```python
from build123d import *

# Parameters (mm, degrees)
SKETCH1_R           = 73.66
BOSS_EXTRUDE1_DEPTH = 0.635
BOSS_EXTRUDE2_START = 52.324
SKETCH2_R           = 73.66
SKETCH2_R_2         = 73.025
BOSS_EXTRUDE2_DEPTH = 52.324
FILLET1_R           = 2.54


with BuildPart() as part:
    # Sketch1 → Boss-Extrude1 (new body)
    with BuildSketch(Plane.XY):
        Circle(SKETCH1_R)
    extrude(amount=BOSS_EXTRUDE1_DEPTH)

    # Sketch2 → Boss-Extrude2 (add)
    with BuildSketch(Plane(origin=(0, 0, 0), x_dir=(-1, 0, 0), z_dir=(0, 0, -1)).offset(BOSS_EXTRUDE2_START)):
        Circle(SKETCH2_R)
        Circle(SKETCH2_R_2, mode=Mode.SUBTRACT)
    extrude(amount=-BOSS_EXTRUDE2_DEPTH)

    # Fillet1
    fillet1_edges = [part.edges().sort_by_distance(p)[0] for p in [
        (-73.66, 0, 0.635),
    ]]
    fillet(fillet1_edges, radius=FILLET1_R)


solid = part.part
```
The listing builds one solid part. Answer for the finished solid, in the listing's coordinates (mm). A direction names the side the tool comes from. Round coordinates to 2 decimals unless told otherwise and drop trailing zeros. Order: outer loops, then holes, each group sorted by start corner. A loop starts at its lowest first (then second) coordinate and runs counter-clockwise, first axis right, second up. Notation, with made-up numbers: (-18, 54) -> (32, 54) arc R15 cw to (32, 65) -> close; hole circle Ø9 at (-39.75, 34). An arc over 180 degrees is marked (long way). Answer as CSV lines item,"result". Start each with the question number.
(1) For a pull along Y with two mould halves and no side action, classify faces 3 (the face through (-1, 1, 0)), 4 (the face through (-1, 1, 0.635)), 5 (the face through (58.454, -44.821, -27.467)) as +Y half, -Y half, draft (parallel to the pull), parting line (faces both ways), or undercut.
(2) Flat-ended cylindrical pins translate along their axes: pin 1 Ø2 at (x, z) = (-42.5, -17.5) entering from -Y; pin 2 Ø4 at (y, z) = (55.5, -38) entering from +X; pin 3 Ø1.5 at (x, z) = (0.5, -45) entering from +Y. Find the tip coordinate at first contact, or state that the pin passes through.
(3) The part is cut by section A-A (z = -26). Determine the outline of the cut face in (x, y) (3 decimals), then the cut area to 3 significant figures.
(4) A tool of negligible diameter and unlimited length cuts with its end or side. For faces 1 (the face through (16.7, 71.3, -52.324)), 2 (the face through (-69.653, 21.935, -26.528)), from which of +Z, -Z, +X, -X, +Y, -Y can it reach the whole face along a straight path? Write none if from no direction.
(5) Find the intervals of material crossed by probe 1 along Y at (x, z) = (0, -33.5) (3 decimals); probe 2 along Z at (x, y) = (22, -33) (3 decimals); probe 3 along X at (y, z) = (-41.5, -19.5), in increasing order. Write a range as from..to.
Evaluation:
1,face 3,"undercut"
1,face 4,"draft"
1,face 5,"parting line"
2,pin 1,"y = -60.86"
2,pin 2,"x = 50.63"
2,pin 3,"y = 73.66"
3,outline,"circle Ø147.32 at (0, 0); hole circle Ø146.05 at (0, 0)"
3,area,"293 mm²"
4,face 1,"-Z, +X, -X, +Y, -Y"
4,face 2,"-Z"
5,probe 1,"-73.66..-73.025, 73.025..73.66"
5,probe 2,"0..0.635"
5,probe 3,"-60.86..-60.09, 60.09..60.86"
